```python
from build123d import *

# Parameters (mm, degrees)
SCHIZZO1_R                   = 4.5
ESTRUSIONE_ESTRUSIONE1_DEPTH = 1.5
SCHIZZO2_R                   = 4
ESTRUSIONE_ESTRUSIONE2_DEPTH = 8


with BuildPart() as part:
    # Schizzo1 → Estrusione-Estrusione1 (new body)
    with BuildSketch(Plane(origin=(0, 0, 0), x_dir=(1, 0, 0), z_dir=(0, 1, 0))):
        with BuildLine():
            Line((10, 0), (249, 0))
            ThreePointArc((249, 0), (256.071067812, 2.928932188), (259, 10))
            Line((259, 10), (259, 120))
            ThreePointArc((259, 120), (256.071067812, 127.071067812), (249, 130))
            Line((249, 130), (10, 130))
            ThreePointArc((10, 130), (2.928932188, 127.071067812), (0, 120))
            Line((0, 120), (0, 10))
            ThreePointArc((0, 10), (2.928932188, 2.928932188), (10, 0))
        make_face()
        with Locations(Location((9, 65, 0), (0, 0, 270))):
            Circle(SCHIZZO1_R, mode=Mode.SUBTRACT)
        with Locations(Location((250, 65, 0), (0, 0, 90))):
            Circle(SCHIZZO1_R, mode=Mode.SUBTRACT)
    extrude(amount=ESTRUSIONE_ESTRUSIONE1_DEPTH)

    # Schizzo2 → Estrusione-Estrusione2 (add)
    # profile 1 of 2: a face of its own
    with BuildSketch(Plane(origin=(0, 1.5, 0), x_dir=(-1, 0, 0), z_dir=(0, 1, 0))):
        Polygon((-9, -57.494446501), (-15.5, -61.24722325), (-15.5, -68.75277675), (-9, -72.505553499), (-2.5, -68.75277675), (-2.5, -61.24722325), align=None)
        with Locations(Location((-9, -65, 0), (0, 0, 270))):
            Circle(SCHIZZO2_R, mode=Mode.SUBTRACT)
    # profile 2 of 2: a face of its own
    with BuildSketch(Plane(origin=(0, 1.5, 0), x_dir=(-1, 0, 0), z_dir=(0, 1, 0))):
        Polygon((-256.5, -61.24722325), (-250, -57.494446501), (-243.5, -61.24722325), (-243.5, -68.75277675), (-250, -72.505553499), (-256.5, -68.75277675), align=None)
        with Locations(Location((-250, -65, 0), (0, 0, 90))):
            Circle(SCHIZZO2_R, mode=Mode.SUBTRACT)
    extrude(amount=ESTRUSIONE_ESTRUSIONE2_DEPTH)


solid = part.part
```
CAD build for the part. Positions are in the model's coordinates, mm. A direction names the side the tool comes from. Coordinates: 2 decimals unless noted, no trailing zeros. Write each loop counter-clockwise with the first axis right and the second up, starting at its lowest first coordinate (ties: lowest second). Pieces come first, ordered by that corner, then holes. Notation, with made-up numbers: (-12.5, 4.25) -> (27.5, 4.25) arc R23 ccw to (27.5, 38.25) -> close; hole circle Ø8 at (84, -19.75). An arc over 180 degrees is marked (long way). Use CSV: the item, a comma, the result in double quotes. Start each with the question number.
Item 1: Band-saw the part on A-A, the plane y = 6.5. Write the cut outline in (x, z).
Item 2: Band-saw the part on B-B, the plane z = -65. Write the cut outline in (x, y).
Item 3: Tool access for faces 4 (the flat face through (5.8, 5.44, -70.66)), 5 (the flat face through (246.7, 5.4, -70.6)), 6 (the flat face through (243.5, 5, -65)), 7 (the flat face through (12.2, 5.44, -59.34)): list every direction of +Z, -Z, +X, -X, +Y, -Y with a clear straight run to the whole face (end or side of a thin tool).
Item 4: Band-saw the part on C-C, the plane x = 163. Write the cut outline in (y, z), plus the area to 3 significant figures.
Item 5: Two-plate mould, pull along X, no slides. Class faces 1 (the flat face through (128, 0, -66)), 2 (the cylindrical face through (10.352, 0.74, -60.708)), 3 (the cylindrical face through (255.99, 0.74, -2.85)): +X half, -X half, draft (parallel to the pull), parting line (faces both ways), or undercut.
Item 6: Wall check: probe 1 along X at (y, z) = (5.5, -65); probe 2 along X at (y, z) = (0.65, -65); probe 3 along Y at (x, z) = (31.5, -50.5). Give the ranges that are in metal, low to high.
Item 7: Drop a flat-ended pin along its axis: P1, Ø4, axis at y = 5, z = -66, coming from the +X side. Give the stop position or say it passes through.
Item 8: Band-saw the part on D-D, the plane z = -99.5. Write the cut outline in (x, y), plus the area to 4 significant figures.
Response values:
1,outline,"(2.5, -68.75) -> (9, -72.51) -> (15.5, -68.75) -> (15.5, -61.25) -> (9, -57.49) -> (2.5, -61.25) -> close; (243.5, -68.75) -> (250, -72.51) -> (256.5, -68.75) -> (256.5, -61.25) -> (250, -57.49) -> (243.5, -61.25) -> close; hole circle Ø8 at (9, -65); hole circle Ø8 at (250, -65)"
2,outline,"(0, 0) -> (4.5, 0) -> (4.5, 1.5) -> (5, 1.5) -> (5, 9.5) -> (2.5, 9.5) -> (2.5, 1.5) -> (0, 1.5) -> close; (13, 1.5) -> (13.5, 1.5) -> (13.5, 0) -> (245.5, 0) -> (245.5, 1.5) -> (246, 1.5) -> (246, 9.5) -> (243.5, 9.5) -> (243.5, 1.5) -> (15.5, 1.5) -> (15.5, 9.5) -> (13, 9.5) -> close; (254, 1.5) -> (254.5, 1.5) -> (254.5, 0) -> (259, 0) -> (259, 1.5) -> (256.5, 1.5) -> (256.5, 9.5) -> (254, 9.5) -> close"
3,face 4,"-Z, -X, +Y"
3,face 5,"-Z, +Y"
3,face 6,"+Z, -Z, +Y"
3,face 7,"+Z, +Y"
4,outline,"(0, -130) -> (1.5, -130) -> (1.5, 0) -> (0, 0) -> close"
4,area,"195 mm2"
5,face 1,"draft"
5,face 2,"undercut"
5,face 3,"+X half"
6,probe 1,"x = 2.5 to 5, 13 to 15.5, 243.5 to 246, 254 to 256.5"
6,probe 2,"x = 0 to 4.5, 13.5 to 245.5, 254.5 to 259"
6,probe 3,"y = 0 to 1.5"
7,P1,"stops at x = 256.5"
8,outline,"(0, 0) -> (259, 0) -> (259, 1.5) -> (0, 1.5) -> close"
8,area,"388.5 mm2"
